Design review of the part built by this model. Coordinates are the model's own, in mm. A direction names the side the tool comes from. Coordinates: 2 decimals unless noted, no trailing zeros. Write each loop counter-clockwise with the first axis right and the second up, starting at its lowest first coordinate (ties: lowest second). Pieces come first, ordered by that corner, then holes.
Q1. Take a section at D-D, the plane x = 17.5. Write out the cut boundary in (y, z), plus the area to 3 significant figures.
Q2. For pin 1 Ø1.5 at (x, z) = (40.5, 6) entering from -Y; pin 2 Ø3 at (x, y) = (-25, 2) entering from -Z; pin 3 Ø5 at (x, z) = (-14, 4) entering from -Y, all flat-tipped, find the tip position at first contact; note any pin that passes through.
Q3. Take a section at C-C, the plane y = -8.5. Write out the cut boundary in (x, z).
Q4. Take a section at A-A, the plane x = -32.5. Write out the cut boundary in (y, z).
Q5. The part is to be moulded in two halves that separate along Z. For faces 4 (the flat face through (-51, -13, 5)), 5 (the flat face through (-15, 1, 10)), 6 (the flat face through (-13.412, 3, 5)), say which applies: released by +Z, released by -Z, zero draft, split by the parting line, or undercut.
Q6. Take a section at B-B, the plane z = 5. Write out the cut boundary in (x, y).
Q7. For faces 1 (the flat face through (-43.412, 3, 5)), 2 (the flat face through (-3.2, 6, 9.4)), 3 (the flat face through (-49.412, -12, 5)), list the 3-axis set-ups (+Z, -Z, +X, -X, +Y, -Y) from which the entire face can be reached by the end or side of a thin tool; tool diameter is ignored.
Q8. For L1, parallel to X at y = 4.1, z = 5; L2, parallel to Z at x = -41, y = 0.5; L3, parallel to X at y = 5, z = 4, list the stretches that pass through material, from the lowest coordinate up.
from build123d import *

# Parameters (mm, degrees)
SALIENTE_EXTRUIR1_DEPTH = 10
CROQUIS4_R              = 4
CROQUIS4_W              = 30
CROQUIS4_H              = 3
CORTAR_EXTRUIR1_DEPTH   = 10


with BuildPart() as part:
    # Croquis2 → Saliente-Extruir1 (new body)
    with BuildSketch(Plane.XY):
        Polygon((-43.412140575, 0), (35.587859425, 0), (38.587859425, 0), (38.587859425, -10), (41.587859425, -10), (41.587859425, -13), (44.587859425, -13), (44.587859425, 6), (-52.412140575, 6), (-52.412140575, -13), (-49.412140575, -13), (-49.412140575, -10), (-46.412140575, -10), (-46.412140575, 0), align=None)
    extrude(amount=SALIENTE_EXTRUIR1_DEPTH)

    # Croquis4 → Cortar-Extruir1 (cut)
    with BuildSketch(Plane(origin=(0, 6, 0), x_dir=(1, 0, 0), z_dir=(0, 1, 0))):
        with Locations((-3.912140575, -5)):
            Circle(CROQUIS4_R)
        with Locations((-28.412140575, -5)):
            Rectangle(CROQUIS4_W, CROQUIS4_H)
    extrude(amount=-CORTAR_EXTRUIR1_DEPTH, mode=Mode.SUBTRACT)


solid = part.part
Responses:
1. outline: (0, 0) - (6, 0) - (6, 10) - (0, 10) - close
1. area: 60.0 mm2
2. pin 1: stops at y = -10
2. pin 2: stops at z = 0
2. pin 3: stops at y = 0
3. outline: (-52.41, 0) - (-46.41, 0) - (-46.41, 10) - (-52.41, 10) - close; (38.59, 0) - (44.59, 0) - (44.59, 10) - (38.59, 10) - close
4. outline: (0, 0) - (6, 0) - (6, 3.5) - (0, 3.5) - close; (0, 6.5) - (6, 6.5) - (6, 10) - (0, 10) - close
5. face 4: zero draft
5. face 5: released by +Z
5. face 6: undercut
6. outline: (-52.41, -13) - (-49.41, -13) - (-49.41, -10) - (-46.41, -10) - (-46.41, 0) - (-43.41, 0) - (-43.41, 6) - (-52.41, 6) - close; (-13.41, 0) - (-7.91, 0) - (-7.91, 6) - (-13.41, 6) - close; (0.09, 0) - (38.59, 0) - (38.59, -10) - (41.59, -10) - (41.59, -13) - (44.59, -13) - (44.59, 6) - (0.09, 6) - close
7. face 1: +Y, -Y
7. face 2: +Z, -Z, +X, -X, +Y
7. face 3: +Z, -Z, -Y
8. L1: x = -52.41 to -43.41, -13.41 to -7.91, 0.09 to 44.59
8. L2: z = 0 to 3.5, 6.5 to 10
8. L3: x = -52.41 to -43.41, -13.41 to -7.79, -0.04 to 44.59
